Design review of the part built by this model. Coordinates are the model's own, in mm. Face numbers are marked on the shaded views. Coordinates: 2 decimals unless noted, no trailing zeros. Loops run counter-clockwise (first coordinate to the right, second up) from the corner with the lowest first, then second, coordinate; pieces in that order, holes last. Notation, with made-up numbers: M 14.5,-10.5 L 50.5,-10.5 A30 ccw 50.5,11.5 Z; hole C 78,78.5 d7. An arc over 180 degrees is marked long. Put each result on its own line as item: value. Start each with the question number.
(1) The part is to be moulded in two halves that separate along X. For the marked faces 1, 2 and 3, say which applies: +X half, -X half, draft (parallel to the pull), parting line (faces both ways), or undercut.
(2) Take a section at C-C, the plane y = 22. Give the boundary of the cut face in (x, z).
(3) Clearance check with flat-ended pins moving along their axes: pin 1 (5 mm diameter, centred on x = -9.5, z = 27.5, fed in from -Y); pin 2 (5 mm diameter, centred on y = 35.5, z = 25, fed in from +X); pin 3 (12 mm diameter, centred on x = -7, z = 25.5, fed in from -Y). State where each tip first meets the part, or that it passes through.
(4) Take a section at B-B, the plane y = 0. Give the boundary of the cut face in (x, z), then the cut area to 3 significant figures.
(5) For probe 1 along Y at (x, z) = (-1.5, 28); probe 2 along X at (y, z) = (15, 22); probe 3 along X at (y, z) = (10, 22.25), list the stretches that pass through material, from the lowest coordinate up. Write a range as [from, to].
(6) Take a section at D-D, the plane z = 40.5. Give the boundary of the cut face in (x, y).
(7) Take a section at A-A, the plane x = 0. Give the boundary of the cut face in (y, z).
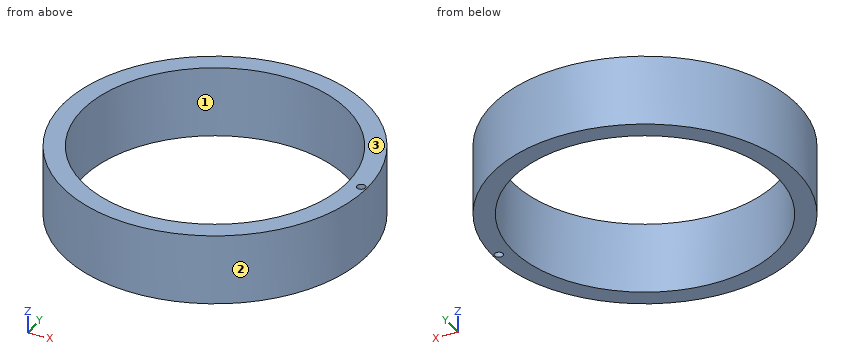
```python
from build123d import *

# Parameters (mm, degrees)
CYLINDER1142_R     = 1.5
CYLINDER1142_DEPTH = 50
TUBE102_R          = 54
TUBE102_R_2        = 47
TUBE102_DEPTH      = 25


with BuildPart() as obj1:
    # Cylinder1142 → Cylinder1142 (new body)
    with BuildSketch(Plane(origin=(52, 0, 0), x_dir=(1, 0, 0), z_dir=(0, 0, 1))):
        Circle(CYLINDER1142_R)
    extrude(amount=CYLINDER1142_DEPTH)


with BuildPart() as obj2:
    # Tube102 → Tube102 (new body)
    with BuildSketch(Plane.XY.offset(20)):
        Circle(TUBE102_R)
        Circle(TUBE102_R_2, mode=Mode.SUBTRACT)
    extrude(amount=TUBE102_DEPTH)

    # Cut: cut obj1
    add(obj1.part, mode=Mode.SUBTRACT)


solid = obj2.part
```
Computed values:
1. face 1: undercut
1. face 2: parting line
1. face 3: draft
2. outline: M -49.32,20 L -41.53,20 L -41.53,45 L -49.32,45 Z; M 41.53,20 L 49.32,20 L 49.32,45 L 41.53,45 Z
3. pin 1: stops at y = -53.54
3. pin 2: stops at x = 42.74
3. pin 3: stops at y = -53.99
4. outline: M -54,20 L -47,20 L -47,45 L -54,45 Z; M 47,20 L 50.5,20 L 50.5,45 L 47,45 Z; M 53.5,20 L 54,20 L 54,45 L 53.5,45 Z
4. area: 275 mm^2
5. probe 1: y = [-53.98, -46.98], [46.98, 53.98]
5. probe 2: x = [-51.87, -44.54], [44.54, 51.87]
5. probe 3: x = [-53.07, -45.92], [45.92, 53.07]
6. outline: C 0,0 d108; hole C 0,0 d94; hole C 52,0 d3
7. outline: M -54,20 L -47,20 L -47,45 L -54,45 Z; M 47,20 L 54,20 L 54,45 L 47,45 Z
